Answer from the drawing. Dimensions are ordinates in mm from the lowest x, y and z of the part. A direction names the side the tool comes from. Give positions to 0.01 mm unless a question says otherwise; leave off trailing zeros. Loops run counter-clockwise (first coordinate to the right, second up) from the corner with the lowest first, then second, coordinate; pieces in that order, holes last. Notation, with made-up numbers: M 52,81 L 75,81 A25 cw 75,113 Z; hole C 33.5,87.5 d5. An arc over 180 degrees is marked long. Use a Markdown table: item, result.
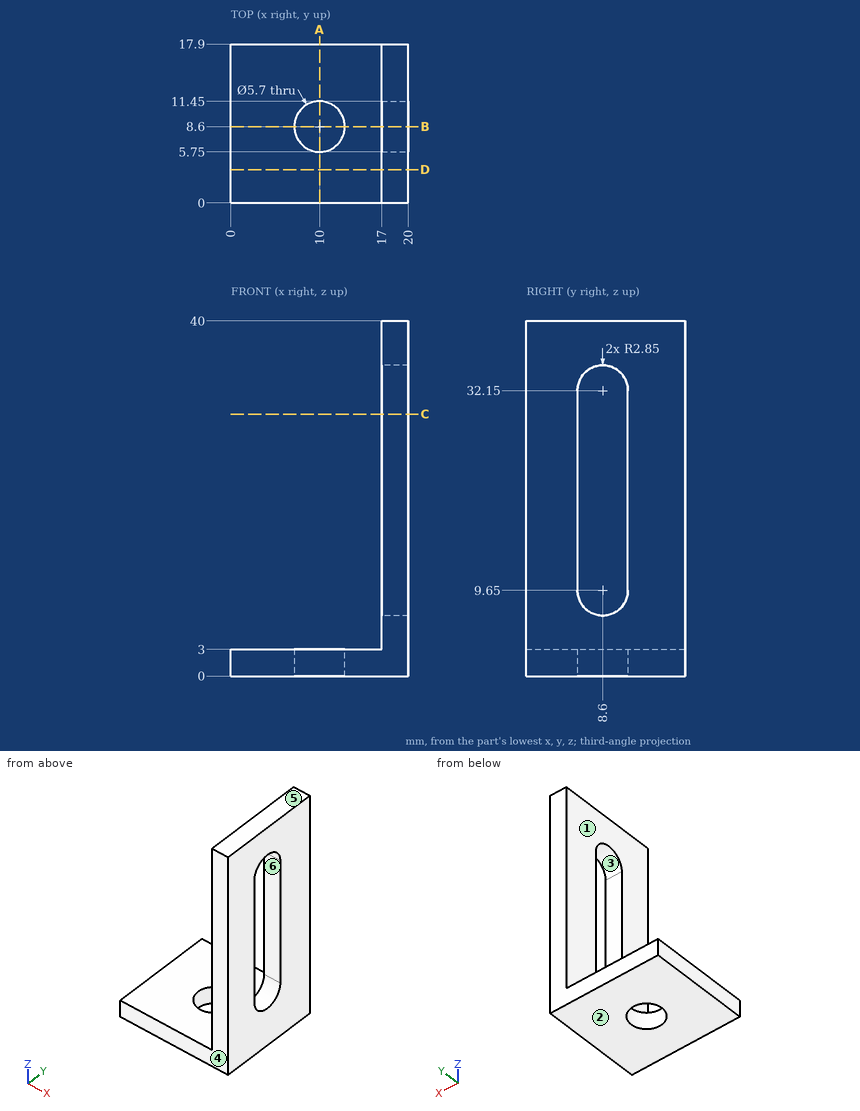
(1) A cutting plane is placed at A-A (x = 10). Write down the section's boundary in (y, z), and give its area (3 significant figures).
Entries:
| item | result |
|---|---|
| outline | M 0,0 L 5.75,0 L 5.75,3 L 0,3 Z; M 11.45,0 L 17.9,0 L 17.9,3 L 11.45,3 Z |
| area | 36.6 mm² |
(2) Given P1, Ø8, axis at y = 3.5, z = 35, coming from the -X side; P2, Ø5, axis at x = 9, y = 8.5, coming from the +Z side, each flat-ended and moving along its own axis, determine where each tip first touches the part or whether it passes through.
Entries:
| item | result |
|---|---|
| P1 | stops at x = 17 |
| P2 | stops at z = 3 |
(3) Which of the six approach directions +Z, -Z, +X, -X, +Y, -Y give full straight-line access (tool end or side, diameter ignored) to the marked faces 1, 2 and 3?
Entries:
| item | result |
|---|---|
| face 1 | +Z, -X, +Y, -Y |
| face 2 | -Z, +X, -X, +Y, -Y |
| face 3 | +X, -X |
(4) A cutting plane is placed at D-D (y = 3.75). Write down the section's boundary in (x, z).
Entries:
| item | result |
|---|---|
| outline | M 0,0 L 20,0 L 20,40 L 17,40 L 17,3 L 0,3 Z |
(5) A cutting plane is placed at B-B (y = 8.6). Write down the section's boundary in (x, z), and give its area (3 significant figures).
Entries:
| item | result |
|---|---|
| outline | M 0,0 L 7.15,0 L 7.15,3 L 0,3 Z; M 12.85,0 L 20,0 L 20,6.8 L 17,6.8 L 17,3 L 12.85,3 Z; M 17,35 L 20,35 L 20,40 L 17,40 Z |
| area | 69.3 mm² |
(6) A cutting plane is placed at C-C (z = 29.5). Write down the section's boundary in (x, y), and give its area (3 significant figures).
Entries:
| item | result |
|---|---|
| outline | M 17,0 L 20,0 L 20,5.75 L 17,5.75 Z; M 17,11.45 L 20,11.45 L 20,17.9 L 17,17.9 Z |
| area | 36.6 mm² |
(7) Consider probe 1 along Y at (x, z) = (10, 2); probe 2 along Z at (x, y) = (7.25, 14.5); probe 3 along Y at (x, z) = (18, 8). Determine where each line is inside the solid, lowest interval first. Write a range as [from, to].
Entries:
| item | result |
|---|---|
| probe 1 | y = [0, 5.75], [11.45, 17.9] |
| probe 2 | z = [0, 3] |
| probe 3 | y = [0, 6.28], [10.92, 17.9] |
(8) The mould has two halves that part along Y. Classify the marked faces 4, 5 and 6: released by +Y, released by -Y, zero draft, split by the parting line, or undercut.
Entries:
| item | result |
|---|---|
| face 4 | released by -Y |
| face 5 | zero draft |
| face 6 | undercut |
